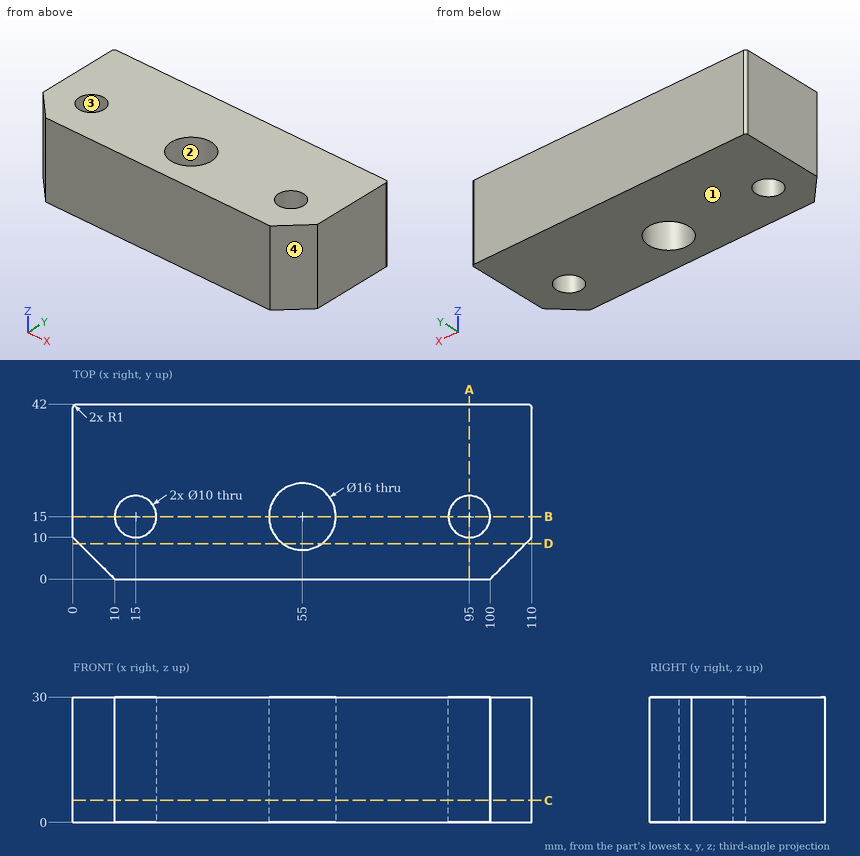
For this review, use the dimensioned drawing (mm, ordinates from the lowest corner) and the shaded views. Give positions to 0.01 mm unless a question says otherwise; leave off trailing zeros. Order: outer loops, then holes, each group sorted by start corner. A loop starts at its lowest first (then second) coordinate and runs counter-clockwise, first axis right, second up.
1. Add section D-D, the plane y = 8.5. State the section outline as (x, z) points, then the cut area to 3 significant figures.
Solution:
outline: (1.5, 0) - (50.34, 0) - (50.34, 30) - (1.5, 30) - close; (59.66, 0) - (108.5, 0) - (108.5, 30) - (59.66, 30) - close
area: 2,930 mm2
2. Mouldability with a two-part tool opening along Y and no side actions: class the marked faces 1, 2, 3 and 4 as +Y half, -Y half, draft (parallel to the pull), parting line (faces both ways), or undercut.
Solution:
face 1: draft
face 2: undercut
face 3: undercut
face 4: -Y half
3. Add section B-B, the plane y = 15. State the section outline as (x, z) points, then the cut area to 3 significant figures.
Solution:
outline: (0, 0) - (10, 0) - (10, 30) - (0, 30) - close; (20, 0) - (47, 0) - (47, 30) - (20, 30) - close; (63, 0) - (90, 0) - (90, 30) - (63, 30) - close; (100, 0) - (110, 0) - (110, 30) - (100, 30) - close
area: 2,220 mm2
4. For pin 1 Ø2 at (y, z) = (6.5, 10.5) entering from -X; pin 2 Ø5 at (y, z) = (5, 8) entering from +X, all flat-tipped, find the tip position at first contact; note any pin that passes through.
Solution:
pin 1: stops at x = 2.5
pin 2: stops at x = 107.5
5. To check wall thickness, follow L1, parallel to Y at x = 55, z = 14.25; L2, parallel to X at y = 13, z = 17.25; L3, parallel to X at y = 16.5, z = 14.25. State the ranges of each line that lie inside material, in increasing order.
Solution:
L1: y = 0 to 7, 23 to 42
L2: x = 0 to 10.42, 19.58 to 47.25, 62.75 to 90.42, 99.58 to 110
L3: x = 0 to 10.23, 19.77 to 47.14, 62.86 to 90.23, 99.77 to 110
6. Add section C-C, the plane z = 5.25. State the section outline as (x, y) points.
Solution:
outline: (0, 10) - (10, 0) - (100, 0) - (110, 10) - (110, 41) arc R1 ccw to (109, 42) - (1, 42) arc R1 ccw to (0, 41) - close; hole circle Ø10 at (15, 15); hole circle Ø16 at (55, 15); hole circle Ø10 at (95, 15)
7. Add section A-A, the plane x = 95. State the section outline as (y, z) points, then the cut area to 3 significant figures.
Solution:
outline: (0, 0) - (10, 0) - (10, 30) - (0, 30) - close; (20, 0) - (42, 0) - (42, 30) - (20, 30) - close
area: 960 mm2
